Can you work these out from the model? Positions are in its coordinate system, mm. A direction names the side the tool comes from. Coordinates: 2 decimals unless noted, no trailing zeros. Loops run counter-clockwise (first coordinate to the right, second up) from the corner with the lowest first, then second, coordinate; pieces in that order, holes last. Notation, with made-up numbers: (11.5, -8.75) -> (67.5, -8.75) arc R18 cw to (67.5, 9.25) -> close; hole circle Ø6 at (-18, 70.25). An arc over 180 degrees is marked (long way). Put each result on its own line as item: value. Start each with the question number.
Item 1: If we section it at B-B on x = 0.75: Please give me the cut outline in (y, z), plus the area to 3 significant figures.
Item 2: If we section it at C-C on z = -0.25: Please give me the cut outline in (x, y).
Item 3: If we section it at A-A on y = 2.75: Please give me the cut outline in (x, z).
Item 4: We'd pull the mould along X, two halves only. Please class faces 4 (the flat face through (-1.394, 7.395, 2.37)), 5 (the flat face through (0, 9, 0)), 6 (the flat face through (-1.3, 15, 1.4)): pulls with the +X half, pulls with the -X half, needs draft (parallel to the pull), parting line crosses it, or undercut.
Item 5: Will this pin go through, and if not, where does the flat tip stop? P1, Ø3, axis at x = 1, z = 1.5, coming from the -Y side.
Item 6: Please list where these lines run through material, in increasing order: L1, parallel to X at y = 13.8, z = 0; L2, parallel to Y at x = 0.65, z = -0.25; L3, parallel to Y at x = 0.4, z = -1.75. Write a range as from..to.
Item 7: If we section it at D-D on x = -2.15: Please give me the cut outline in (y, z), plus the area to 3 significant figures.
Item 8: For faces 1 (the cylindrical face through (-1.5, 12.04, -0.07)), 2 (the flat face through (1.394, 7.395, -2.37)), 3 (the flat face through (-1.3, 0, 1.4)), which set-ups out of +Z, -Z, +X, -X, +Y, -Y let a thin tool reach every point of the face, with its end or its side?
```python
from build123d import *

# Parameters (mm, degrees)
SALIENTE_EXTRUIR1_DEPTH = 15
CROQUIS2_R              = 1.5
SALIENTE_EXTRUIR2_DEPTH = 6
CROQUIS3_R              = 1.5
CORTAR_EXTRUIR1_DEPTH   = 6


with BuildPart() as part:
    # Croquis1 → Saliente-Extruir1 (new body)
    with BuildSketch(Plane(origin=(0, 0, 0), x_dir=(1, 0, 0), z_dir=(0, 1, 0))):
        Polygon((0, 3.175426481), (-2.75, 1.58771324), (-2.75, -1.58771324), (0, -3.175426481), (2.75, -1.58771324), (2.75, 1.58771324), align=None)
    extrude(amount=SALIENTE_EXTRUIR1_DEPTH)

    # Croquis2 → Saliente-Extruir2 (add)
    with BuildSketch(Plane.XZ):
        Circle(CROQUIS2_R)
    extrude(amount=SALIENTE_EXTRUIR2_DEPTH)

    # Croquis3 → Cortar-Extruir1 (cut)
    with BuildSketch(Plane(origin=(0, 15, 0), x_dir=(1, 0, 0), z_dir=(0, 1, 0))):
        Circle(CROQUIS3_R)
    extrude(amount=-CORTAR_EXTRUIR1_DEPTH, mode=Mode.SUBTRACT)


solid = part.part
```
Solutions:
1. outline: (-6, -1.3) -> (0, -1.3) -> (0, -2.74) -> (15, -2.74) -> (15, -1.3) -> (9, -1.3) -> (9, 1.3) -> (15, 1.3) -> (15, 2.74) -> (0, 2.74) -> (0, 1.3) -> (-6, 1.3) -> close
1. area: 82.3 mm^2
2. outline: (-2.75, 0) -> (-1.48, 0) -> (-1.48, -6) -> (1.48, -6) -> (1.48, 0) -> (2.75, 0) -> (2.75, 15) -> (1.48, 15) -> (1.48, 9) -> (-1.48, 9) -> (-1.48, 15) -> (-2.75, 15) -> close
3. outline: (-2.75, -1.59) -> (0, -3.18) -> (2.75, -1.59) -> (2.75, 1.59) -> (0, 3.18) -> (-2.75, 1.59) -> close
4. face 4: pulls with the -X half
4. face 5: undercut
4. face 6: needs draft
5. P1: y = -6
6. L1: -2.75..-1.5, 1.5..2.75
6. L2: -6..9
6. L3: 0..15
7. outline: (0, -1.93) -> (15, -1.93) -> (15, 1.93) -> (0, 1.93) -> close
7. area: 58.0 mm^2
8. face 1: +Y
8. face 2: -Z, +X, +Y, -Y
8. face 3: -Y
